Source: three-view drawing plus pictorial views. Frame: mm from the lowest corner of the part. A direction names the side the tool comes from. Give positions to 0.01 mm unless a question says otherwise; leave off trailing zeros. Write each loop counter-clockwise with the first axis right and the second up, starting at its lowest first coordinate (ties: lowest second). Pieces come first, ordered by that corner, then holes.
Q1. Line query: L1, parallel to X at y = 17, z = 1; L2, parallel to X at y = 5.5, z = 8; L3, parallel to Y at x = 44, z = 7.5. Output: solid intervals per line, ascending.
Q2. Draft query along Y for the marked faces 3, 4, 5 and 6. Return one class per face: pulls with the +Y half, pulls with the -Y half, needs draft (parallel to the pull), parting line crosses it, or undercut.
Q3. Reachability of the marked faces 1 and 2 from +Z, -Z, +X, -X, +Y, -Y: full face, straight path, thin tool, end or side. Return the list, or none.
Q4. Cut plane C-C on z = 7.5. Return the cut outline in (x, y), plus the area to 3 significant figures.
Q5. Pin query (flat end, axial travel): pin 1 (1.5 mm diameter, centred on x = 23, y = 9.5, fed in from -Z). Return the tip coordinate at first contact, or that it passes through.
Q6. Cut plane A-A on x = 12.5. Return the cut outline in (y, z), plus the area to 3 significant figures.
Q7. Cut plane B-B on y = 34.5. Return the cut outline in (x, z).
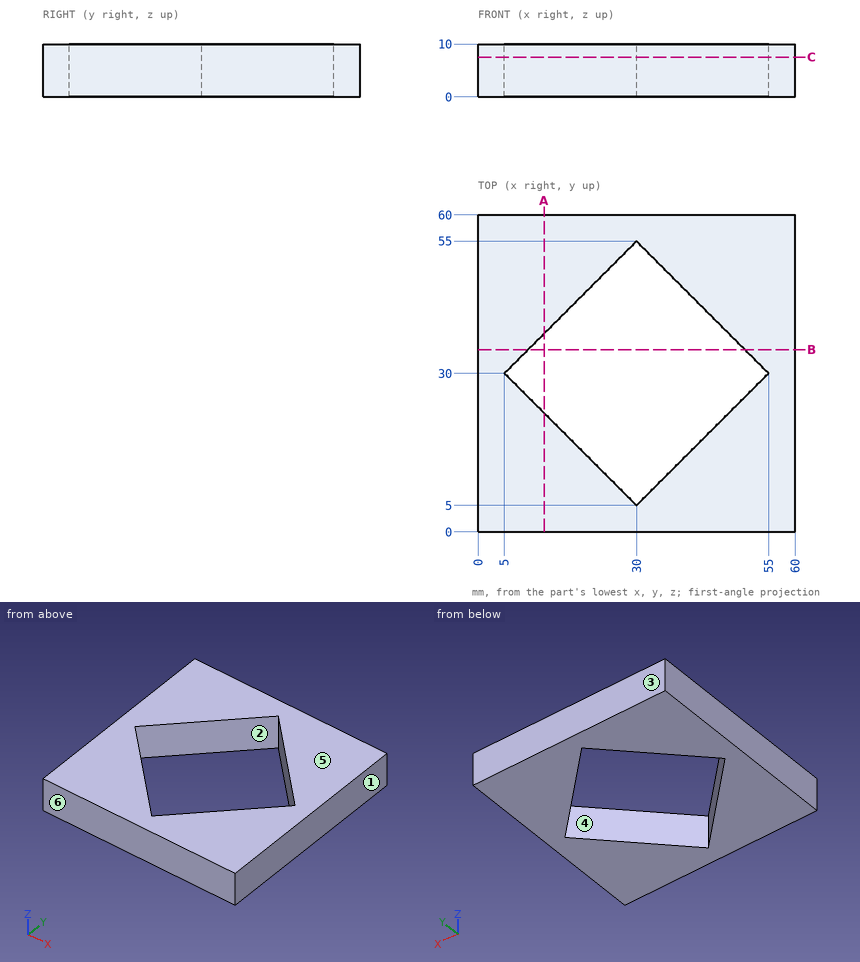
Data:
1. L1: x = 0 to 18, 42 to 60
1. L2: x = 0 to 29.5, 30.5 to 60
1. L3: y = 0 to 19, 41 to 60
2. face 3: pulls with the +Y half
2. face 4: undercut
2. face 5: needs draft
2. face 6: pulls with the -Y half
3. face 1: +Z, -Z, +X, +Y, -Y
3. face 2: +Z, -Z
4. outline: (0, 0) - (60, 0) - (60, 60) - (0, 60) - close; hole (5, 30) - (30, 5) - (55, 30) - (30, 55) - close
4. area: 2,350 mm2
5. pin 1: stops at z = 0
6. outline: (0, 0) - (22.5, 0) - (22.5, 10) - (0, 10) - close; (37.5, 0) - (60, 0) - (60, 10) - (37.5, 10) - close
6. area: 450 mm2
7. outline: (0, 0) - (9.5, 0) - (9.5, 10) - (0, 10) - close; (50.5, 0) - (60, 0) - (60, 10) - (50.5, 10) - close
